from build123d import *

# Parameters (mm, degrees)
F3_DEPTH = 6.35


with BuildPart() as f1:
    # F0 (on Front) → F1 (revolve)
    with BuildSketch(Plane.XZ):
        with BuildLine():
            Line((0, 15.875), (0, 0))
            Line((0, 0), (8.5598, 0))
            ThreePointArc((8.5598, 0), (9.242299, 0.282701), (9.525, 0.9652))
            Line((9.525, 0.9652), (9.525, 11.742871))
            ThreePointArc((9.525, 11.742871), (9.244663, 12.419663), (8.567871, 12.7))
            Line((8.567871, 12.7), (5.08, 12.7))
            Line((5.08, 12.7), (5.08, 14.917871))
            ThreePointArc((5.08, 14.917871), (4.799663, 15.594663), (4.122871, 15.875))
            Line((4.122871, 15.875), (0, 15.875))
        make_face()
    revolve(axis=Axis((0, 0, 7.9375), (0, 0, -1)))

    # F2 (on Front) → F3 (join, symmetric)
    with BuildSketch(Plane.XZ):
        Polygon((9.525, 0), (0, 0), (0, -25.4), (16.51, -25.4), align=None)
    extrude(amount=F3_DEPTH, both=True)

    # F4: F1 across plane


with BuildPart() as f1_1:
    add(f1.part)
    add(f1.part.mirror(Plane.YZ))


solid = f1_1.part
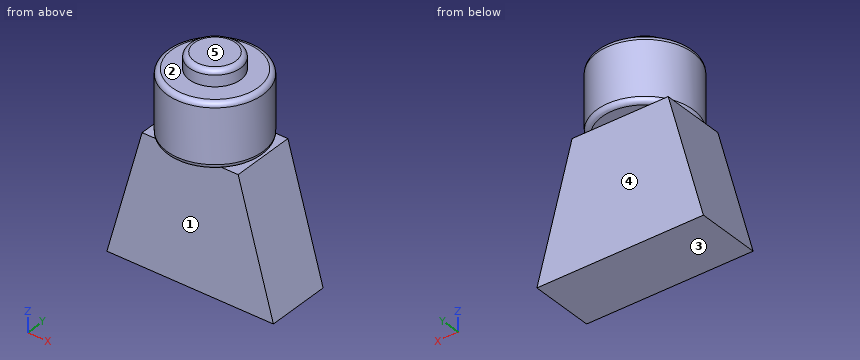
Read the model definition and answer for the solid it produces. Units are mm, in the model's axes. Face numbers are marked on the shaded views. A direction names the side the tool comes from. Round coordinates to 2 decimals unless told otherwise and drop trailing zeros. Loops run counter-clockwise (first coordinate to the right, second up) from the corner with the lowest first, then second, coordinate; pieces in that order, holes last. Notation, with made-up numbers: (-15.5, -33) - (41.5, -33) arc R11 ccw to (41.5, -13) - close; hole circle Ø5 at (34.5, 36.25). An arc over 180 degrees is marked (long way). One line per question, with ' | ' between items. Start each with the question number.
Q1. Flat-ended cylindrical pins translate along their axes: pin 1 (6 mm diameter, centred on y = 5, z = -13.5, fed in from -X); pin 2 (1.5 mm diameter, centred on y = -5.5, z = -11, fed in from -X); pin 3 (1.9 mm diameter, centred on x = -8, y = 3, fed in from +Z). Find the tip coordinate at first contact, or state that the pin passes through.
Q2. Section C-C on x = -10 is taken. Give the vertices of the cut face in (y, z), plus the area to 3 significant figures.
Q3. Section A-A on x = 0 is taken. Give the vertices of the cut face in (y, z) (3 decimals), plus the area to 3 significant figures.
Q4. Section B-B on y = 0 is taken. Give the vertices of the cut face in (x, z) (3 decimals), plus the area to 3 significant figures.
Q5. Find the intervals of material crossed by L1, parallel to Z at x = 8.5, y = 6; L2, parallel to Z at x = 3, y = 7; L3, parallel to Y at x = -11.5, z = -21.5, in increasing order.
Q6. For the marked faces 1, 2, 3, 4 and 5, determine the directions among +Z, -Z, +X, -X, +Y, -Y from which every point of the face is accessible in a straight line to the end or side of a thin tool.
Established:
1) pin 1: x = -14.06 | pin 2: x = -12.76 | pin 3: z = 12.7
2) outline: (-6.35, -25.4) - (6.35, -25.4) - (6.35, -1.73) - (-6.35, -1.73) - close | area: 301 mm²
3) outline: (-9.525, 0.965) arc R0.965 ccw to (-8.56, 0) - (-6.35, 0) - (-6.35, -25.4) - (6.35, -25.4) - (6.35, 0) - (8.56, 0) arc R0.965 ccw to (9.525, 0.965) - (9.525, 11.743) arc R0.957 ccw to (8.568, 12.7) - (5.08, 12.7) - (5.08, 14.918) arc R0.957 ccw to (4.123, 15.875) - (-4.123, 15.875) arc R0.957 ccw to (-5.08, 14.918) - (-5.08, 12.7) - (-8.568, 12.7) arc R0.957 ccw to (-9.525, 11.743) - close | area: 596 mm²
4) outline: (-16.51, -25.4) - (16.51, -25.4) - (9.525, 0) - (8.56, 0) arc R0.965 ccw to (9.525, 0.965) - (9.525, 11.743) arc R0.957 ccw to (8.568, 12.7) - (5.08, 12.7) - (5.08, 14.918) arc R0.957 ccw to (4.123, 15.875) - (-4.123, 15.875) arc R0.957 ccw to (-5.08, 14.918) - (-5.08, 12.7) - (-8.568, 12.7) arc R0.957 ccw to (-9.525, 11.743) - (-9.525, 0.965) arc R0.965 ccw to (-8.56, 0) - (-9.525, 0) - close | area: 934 mm²
5) L1: -25.4 to 0 | L2: 0 to 12.7 | L3: -6.35 to 6.35
6) face 1: -Z, +X, -X, -Y | face 2: +Z | face 3: -Z, +X, -X, +Y, -Y | face 4: -Z, +X, -X, +Y | face 5: +Z, +X, -X, +Y, -Y
